Can you work these out from the drawing? Everything is in mm from the part's minimum corner. A direction names the side the tool comes from. Coordinates: 2 decimals unless noted, no trailing zeros. Loops run counter-clockwise (first coordinate to the right, second up) from the corner with the lowest first, then second, coordinate; pieces in that order, holes last.
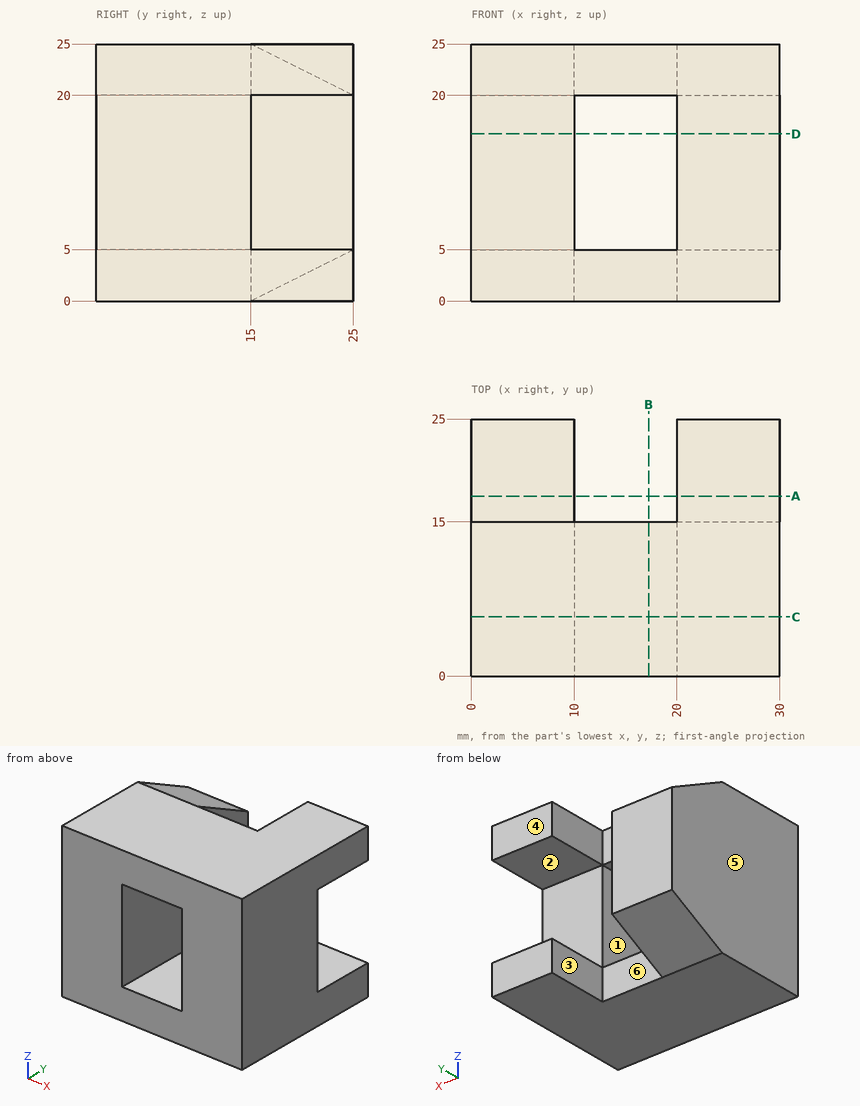
Item 1: I need wall thicknesses on line 1 along Z through (x, y) = (27, 19.5); line 2 along X through (y, z) = (5, 11.5); line 3 along Y through (x, z) = (19.75, 22.5). Which ranges of each line are inside material? Lowest first, please.
Results are:
line 1: z = 0 to 5, 20 to 25
line 2: x = 0 to 10, 20 to 30
line 3: y = 0 to 15
Item 2: On a 3-axis mill with a long thin cutter (end or side, diameter ignored), from which of +Z, -Z, +X, -X, +Y, -Y can I reach the whole of each face in a straight line? I mean the marked faces 1, 2 and 3. Say none if no direction works.
Results are:
face 1: +Y, -Y
face 2: +X, +Y
face 3: +Z, -Z, +Y
Item 3: We'd pull the mould along X, two halves only. Please class the marked faces 4, 5 and 6: +X half, -X half, draft (parallel to the pull), parting line (faces both ways), or undercut.
Results are:
face 4: draft
face 5: -X half
face 6: undercut
Item 4: Suppose I cut it at C-C, the plane y = 5.75. Please give me the cut outline in (x, z), plus the area to 3 significant figures.
Results are:
outline: (0, 0) - (30, 0) - (30, 25) - (0, 25) - close; hole (10, 5) - (20, 5) - (20, 20) - (10, 20) - close
area: 600 mm2
Item 5: Suppose I cut it at B-B, the plane x = 17.25. Please give me the cut outline in (y, z).
Results are:
outline: (0, 0) - (15, 0) - (15, 5) - (0, 5) - close; (0, 20) - (15, 20) - (15, 25) - (0, 25) - close
Item 6: Suppose I cut it at D-D, the plane z = 16.25. Please give me the cut outline in (x, y).
Results are:
outline: (0, 0) - (10, 0) - (10, 25) - (0, 25) - close; (20, 0) - (30, 0) - (30, 15) - (20, 15) - close
Item 7: Suppose I cut it at A-A, the plane y = 17.5. Please give me the cut outline in (x, z), plus the area to 3 significant figures.
Results are:
outline: (0, 1.25) - (10, 1.25) - (10, 23.75) - (0, 23.75) - close; (20, 0) - (30, 0) - (30, 5) - (20, 5) - close; (20, 20) - (30, 20) - (30, 25) - (20, 25) - close
area: 325 mm2
Item 8: I'm going to push flat-ended pins straight in: P1, Ø1.5, axis at x = 7.5, y = 22, coming from the -Z side (3 decimals); P2, Ø4, axis at x = 15, z = 2.5, coming from the +Y side. Where does each tip first touch, or does it pass through?
Results are:
P1: stops at z = 3.125
P2: stops at y = 15
